Geometry: see drawing. Coordinates: mm, zero at the bounding-box minimum. A direction names the side the tool comes from. Give positions to 0.01 mm unless a question says otherwise; leave off trailing zeros. Write each loop counter-clockwise with the first axis right and the second up, starting at its lowest first coordinate (ties: lowest second). Pieces come first, ordered by that corner, then holes. Notation, with made-up numbers: (-7, 33.25) -> (50, 33.25) arc R15 cw to (50, 46.25) -> close; hole circle Ø7 at (-33, -30). An arc over 180 degrees is marked (long way). Answer as a JSON object with one key per item and string values. Group by question number.
Item 1: Section query D-D on y = 5. Return the cut outline in (x, z).
Item 2: Section query C-C on z = 8. Return the cut outline in (x, y) (1 decimal), plus the area to 3 significant figures.
Item 3: Section query B-B on y = 21. Return the cut outline in (x, z).
Item 4: Pull-direction query (X, two-part tool) for the marked faces 3, 4, 5 and 6; classes: pulls with the +X half, pulls with the -X half, needs draft (parallel to the pull), parting line crosses it, or undercut.
Item 5: Ray query, probe 1 along X at (y, z) = (14.5, 14.25); probe 2 along X at (y, z) = (13.5, 1); probe 3 along Z at (x, y) = (11, 29). Return the intervals inside material, ascending. Write a range as from..to.
Item 6: First-contact query: pin 1 Ø0.6 at (y, z) = (14, 0.5) entering from -X; pin 2 Ø9.5 at (x, y) = (18, 18.5) entering from +Z; pin 3 Ø2 at (x, z) = (10, 5) entering from -Y; pin 4 Ø6.5 at (x, y) = (17.32, 8.3) entering from +Z. Flat tips, straight axial feed; report the tip coordinate or a pass-through.
Item 7: Access query for the marked faces 1 and 2. Directions: +Z, -Z, +X, -X, +Y, -Y. A direction counts if a zero-diameter tool reaches every point of the face in a straight line with its end or side. Return the directions, or none.
Item 8: Section query A-A on x = 19. Return the cut outline in (y, z) (1 decimal).
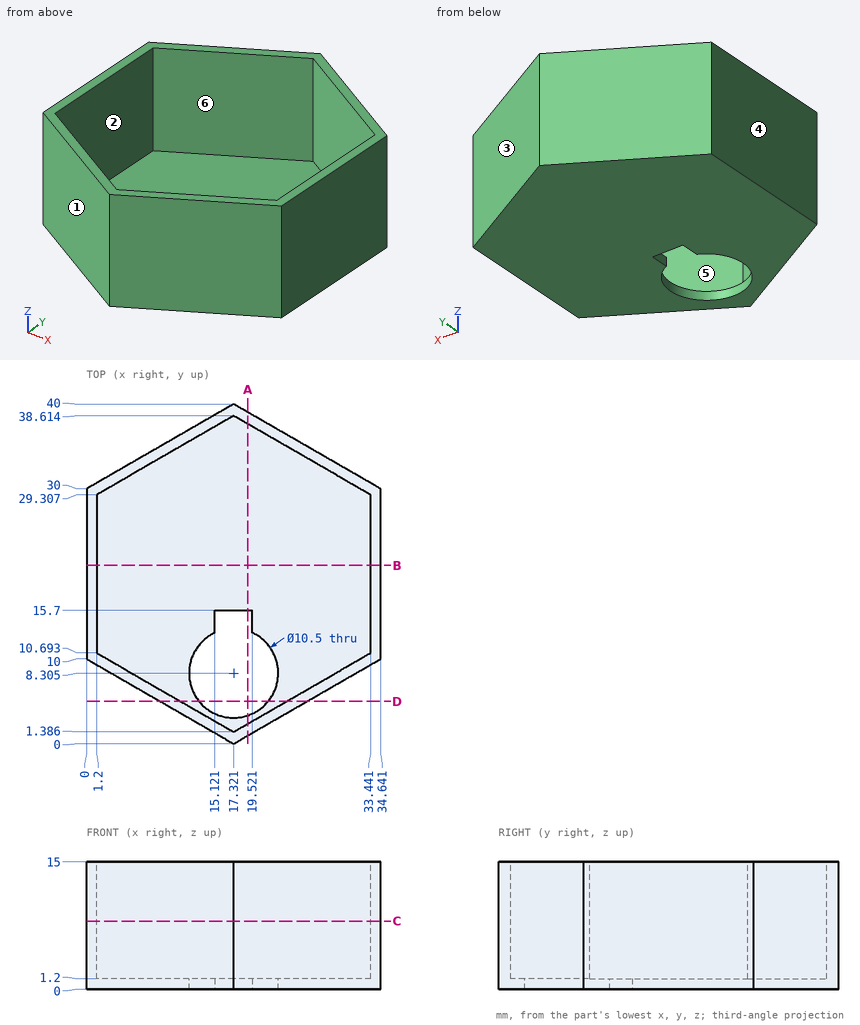
Worked answers:
{
 "1": {"outline": "(8.66, 0) -> (13.24, 0) -> (13.24, 1.2) -> (11.06, 1.2) -> (11.06, 15) -> (8.66, 15) -> close; (21.4, 0) -> (25.98, 0) -> (25.98, 15) -> (23.58, 15) -> (23.58, 1.2) -> (21.4, 1.2) -> close"},
 "2": {"outline": "(0, 10) -> (17.3, 0) -> (34.6, 10) -> (34.6, 30) -> (17.3, 40) -> (0, 30) -> close; hole (1.2, 10.7) -> (17.3, 1.4) -> (33.4, 10.7) -> (33.4, 29.3) -> (17.3, 38.6) -> (1.2, 29.3) -> close", "area": "139 mm^2"},
 "3": {"outline": "(0, 0) -> (34.64, 0) -> (34.64, 15) -> (33.44, 15) -> (33.44, 1.2) -> (1.2, 1.2) -> (1.2, 15) -> (0, 15) -> close"},
 "4": {"face 3": "pulls with the +X half", "face 4": "pulls with the -X half", "face 5": "undercut", "face 6": "undercut"},
 "5": {"probe 1": "0..1.2, 33.44..34.64", "probe 2": "0..15.12, 19.52..34.64", "probe 3": "0..1.2"},
 "6": {"pin 1": "x = 0", "pin 2": "z = 1.2", "pin 3": "y = 3.65", "pin 4": "through"},
 "7": {"face 1": "+Z, -Z, -X, -Y", "face 2": "+Z"},
 "8": {"outline": "(1, 0) -> (3.3, 0) -> (3.3, 1.2) -> (2.4, 1.2) -> (2.4, 15) -> (1, 15) -> close; (15.7, 0) -> (39, 0) -> (39, 15) -> (37.6, 15) -> (37.6, 1.2) -> (15.7, 1.2) -> close"}
}
